Check sheet for the modelled part. Datum: model origin and axes. Units: mm. A direction names the side the tool comes from. Coordinates: 2 decimals unless noted, no trailing zeros. Write each loop counter-clockwise with the first axis right and the second up, starting at its lowest first coordinate (ties: lowest second). Pieces come first, ordered by that corner, then holes. Notation, with made-up numbers: (77, 47.5) -> (108, 47.5) arc R6 cw to (108, 57.5) -> close; hole circle Ø9 at (-28.5, 86.25). An arc over 180 degrees is marked (long way). One line per item, written item: value. Start each with the question number.
1) Sectioned sample at B-B on x = 11.43. Enter the section's corners in (y, z).
2) Gauge pin test, flat ends, axial feed: P1, Ø12, axis at x = 0, y = 0, coming from the -Z side; P2, Ø5.5, axis at x = -23.5, z = -15.5, coming from the -Y side; P3, Ø8, axis at x = -28, y = 19, coming from the +Z side. Record the tip position at first contact, or that the pin passes through.
3) Sectioned sample at C-C on y = -12.7. Enter the section's corners in (x, z).
4) Set-up check for faces 5 (the cylindrical face through (-54.72, 5.79, -8.81)), 6 (the flat face through (-26.513, -15.382, 22.181)), 7 (the flat face through (-35.324, 20.149, -22.269)), 8 (the flat face through (1.27, -24, 16)), 9 (the flat face through (-47.714, 0, -17)): record each of +Z, -Z, +X, -X, +Y, -Y from which the full face is reachable in a straight line by a thin tool's end or side.
5) Sectioned sample at D-D on x = -44.5. Enter the section's corners in (y, z), plus the area to 3 significant figures.
6) Scan lines: line 1 along X through (y, z) = (22, 13); line 2 along Y through (x, z) = (0, -11.25) (3 decimals); line 3 along Z through (x, y) = (20.5, -19). Record each from-to range of solid material in increasing order. Write a range as [from, to].
7) Draft check along Y on faces 1 (the flat face through (-28.354, 20.149, -22.269)), 2 (the cylindrical face through (-31.899, -3.176, -22.269)), 3 (the cylindrical face through (-54.7, 6.4, 8.7)), 4 (the flat face through (0, 0, 25.4)). Enter one of: +Y half, -Y half, draft (parallel to the pull), parting line (faces both ways), or undercut.
8) Sectioned sample at A-A on z = 10.16. Enter the section's corners in (x, y).
Autodesk Inventor part; units mm, degrees
ref_plane "YZ Plane" through (0, 0, 0) normal (1, 0, 0) x (0, 1, 0)
ref_plane "XZ Plane" through (0, 0, 0) normal (0, 1, 0) x (-1, 0, 0)
ref_plane "XY Plane" through (0, 0, 0) normal (0, 0, 1) x (1, 0, 0)
sketch "Sketch1" plane through (0, 0, 0) normal (0, 0, 1) x (1, 0, 0)
  line L0 (-57.8485, 25.4) -> (-51.4985, 25.4)
  line L1 (-51.4985, 25.4) -> (-51.4985, -25.4)
  line L2 (-51.4985, -25.4) -> (-57.8485, -25.4)
  line L3 (-57.8485, -25.4) -> (-57.8485, 25.4)
  line L4 (25.4, 25.4) -> (31.75, 25.4)
  line L5 (31.75, 25.4) -> (31.75, -25.4)
  line L6 (31.75, -25.4) -> (25.4, -25.4)
  line L7 (25.4, -25.4) -> (25.4, 25.4)
  point P0 (0, 0)
  dimension "d0" = 6.35
  dimension "d1" = 50.8
  dimension "d2" = 25.4
  dimension "d3" = 51.4985
  dimension "d4" = 25.4
  dimension "d5" = 25.4
extrude "Extrusion1" add sketch "Sketch1" along normal mid plane 38.1
sketch "Sketch2" plane through (0, 0, 19.05) normal (0, 0, 1) x (1, 0, 0)
  line L0 (-51.4985, 25.4) -> (-57.8485, 25.4)
  line L1 (31.75, -25.4) -> (25.4, -25.4)
  line L2 (-57.8485, 25.4) -> (31.75, 25.4)
  line L3 (31.75, 25.4) -> (31.75, -25.4)
  line L4 (31.75, -25.4) -> (-57.8485, -25.4)
  line L5 (-57.8485, -25.4) -> (-57.8485, 25.4)
  circle A0 centre (0, 0) radius 6.604
  circle A1 centre (-41.3385, 6.35) radius 1.4605
  line L6 (-47.9108, 0) -> (-31.2118, 0) construction
  circle A2 centre (-41.3385, -6.35) radius 1.4605
  line L7 (-51.4985, -25.4) -> (-51.4985, 25.4)
  dimension "d8" = 13.208
  dimension "d40" = 2.921
  dimension "d42" = 19.05
  dimension "d43" = 16.51
  dimension "d44" = 6.35
  dimension "d92" = 6.35
sketch "Sketch3" plane through (0, 0, -19.05) normal (0, 0, -1) x (-1, 0, 0)
  line L0 (-31.75, 25.4) -> (-31.75, -25.4)
  line L1 (51.4985, -25.4) -> (57.8485, -25.4)
  line L2 (-31.75, 25.4) -> (57.8485, 25.4)
  line L3 (57.8485, 25.4) -> (57.8485, -25.4)
  line L4 (57.8485, -25.4) -> (-31.75, -25.4)
  line L5 (-31.75, -25.4) -> (-31.75, 25.4)
  circle A0 centre (0, 0) radius 6.604
  circle A1 centre (-11.43, 0.0226) radius 2.54
  circle A2 centre (-20.2438, 8.7122) radius 1.7907
  line L6 (-13.9699, 0) -> (6.604, 0) construction
  circle A3 centre (-20.2438, -8.7122) radius 1.7907
  circle A4 centre (41.3385, 6.35) radius 1.4605
  line L7 (51.4985, 25.4) -> (51.4985, -25.4)
  circle A5 centre (41.3385, -6.35) radius 1.4605
  dimension "d11" = 13.208
  dimension "d12" = 5.08
  dimension "d13" = 11.43
  dimension "d14" = 3.5814
  dimension "d15" = 20.2438
  dimension "d16" = 8.7122
  dimension "d32" = 2.921
  dimension "d33" = 10.16
  dimension "d34" = 6.35
  dimension "d35" = 6.35
extrude "Extrusion7" add sketch "Sketch2" along normal blind 6.35
extrude "Extrusion6" add sketch "Sketch3" along normal blind 6.35
sketch "Sketch6" plane through (-57.8485, -25.4, 25.4) normal (-1, 0, 0) x (0, 0, 1)
  circle A0 centre (-23.114, 38.1) radius 1.4605
  line L0 (-35.0625, 25.4) -> (-10.5897, 25.4) construction
  line L1 (0, 0) -> (-50.8, 0) construction
  line L2 (0, 50.8) -> (0, 0) construction
  circle A1 centre (-23.114, 12.7) radius 1.4605
  point P0 (-25.4, 25.4)
  dimension "d47" = 2.921
  dimension "d48" = 25.4
  dimension "d49" = 12.7
  dimension "d50" = 23.114
extrude "Extrusion8" cut sketch "Sketch6" against normal up to next
sketch "Sketch8" plane through (-57.8485, 25.4, 25.4) normal (0, 1, 0) x (1, 0, 0)
  line L0 (0, 50.8) -> (0, 0)
  line L1 (0, 21.59) -> (6.35, 21.59)
  line L2 (6.35, 21.59) -> (6.35, 29.21)
  line L3 (6.35, 29.21) -> (0, 29.21)
  line L4 (0, 29.21) -> (0, 21.59)
  line L5 (0, 25.4) -> (6.35, 25.4) construction
  line L6 (89.5985, 0) -> (0, 0)
  line L7 (0, 50.8) -> (89.5985, 50.8)
  line L8 (6.35, 6.35) -> (6.35, 44.45)
  point P0 (57.8485, 25.4)
  point P1 (0, 29.21)
  dimension "d56" = 25.4
  dimension "d57" = 50.8
  dimension "d58" = 7.62
extrude "Extrusion10" cut sketch "Sketch8" against normal through all
sketch "Sketch10" plane through (0, 0, 25.4) normal (0, 0, 1) x (1, 0, 0)
  circle A0 centre (20.2438, -8.7122) radius 1.7907 construction
  circle A1 centre (20.2438, -8.7122) radius 1.7907
  circle A2 centre (20.2438, 8.7122) radius 1.7907 construction
  circle A3 centre (20.2438, 8.7122) radius 1.7907
  circle A4 centre (20.2438, 8.7122) radius 5.08
  circle A5 centre (20.2438, -8.7122) radius 5.08
  point P0 (0, 0)
  dimension "d64" = 10.16
extrude "Extrusion12" cut sketch "Sketch10" against normal blind 25.4 contours A1 | A3 | A4 | A5
sketch "Sketch11" plane through (0, 0, 25.4) normal (0, 0, 1) x (1, 0, 0)
  line L0 (9.525, -9.525) -> (-9.525, -9.525)
  line L1 (-9.525, -9.525) -> (-9.525, 9.525)
  line L2 (-9.525, 9.525) -> (9.525, 9.525)
  line L3 (9.525, 9.525) -> (9.525, -9.525)
  line L4 (9.525, -9.525) -> (-9.525, 9.525) construction
  line L5 (-9.525, -9.525) -> (9.525, 9.525) construction
  point P0 (0, 0)
  dimension "d67" = 19.05
  dimension "d68" = 19.05
extrude "Extrusion13" add sketch "Sketch11" along normal blind 6.35
sketch "Sketch12" plane through (0, 0, -25.4) normal (0, 0, -1) x (-1, 0, 0)
  circle A0 centre (31.8389, -6.35) radius 3.175
  line L0 (57.8485, -25.4) -> (57.8485, 25.4)
  line L1 (34.9338, -5.6412) -> (39.4589, -25.4)
  line L2 (28.744, -5.6412) -> (24.2189, -25.4)
  line L3 (24.2189, -25.4) -> (39.4589, -25.4)
  line L4 (-25.4, -25.4) -> (51.4985, -25.4)
  circle A1 centre (31.8389, 15.24) radius 3.175
  line L5 (57.8485, 25.4) -> (-31.75, 25.4)
  line L6 (28.67, 15.0438) -> (28.0289, 25.4)
  line L7 (51.4985, 25.4) -> (-25.4, 25.4)
  line L8 (35.0078, 15.0438) -> (35.6489, 25.4)
  point P0 (0, 0)
  dimension "d71" = 6.35
  dimension "d72" = 26.0096
  dimension "d73" = 6.35
  dimension "d74" = 15.24
  dimension "d75" = 7.62
  dimension "d78" = 10.16
  dimension "d79" = 7.62
  dimension "d80" = 3.81
extrude "Extrusion14" cut sketch "Sketch12" against normal through all
sketch "Sketch13" plane through (0, 0, -19.05) normal (0, 0, 1) x (1, 0, 0)
  circle A0 centre (0, 0) radius 6.604
  circle A1 centre (0, 0) radius 6.604
  circle A2 centre (0, 0) radius 9.525
  dimension "d81" = 19.05
extrude "Extrusion15" add sketch "Sketch13" along normal blind 12.192
sketch "Sketch14" plane through (31.75, 25.4, 25.4) normal (0, 1, 0) x (1, 0, 0)
  line L0 (-59.7789, 50.8) -> (0, 50.8)
  line L1 (-22.225, 0) -> (-41.275, 0)
  line L2 (-40.64, 50.8) -> (-30.48, 50.8)
  line L3 (-30.48, 50.8) -> (-30.48, 0)
  line L4 (-30.48, 0) -> (-40.64, 0)
  line L5 (-40.64, 0) -> (-40.64, 50.8)
  line L6 (0, 0) -> (0, 50.8)
  point P0 (-31.75, 25.4)
  dimension "d84" = 10.16
  dimension "d85" = 40.64
extrude "Extrusion16" add sketch "Sketch14" against normal blind 3.81
sketch "Sketch15" plane through (0, 0, 19.05) normal (0, 0, -1) x (-1, 0, 0)
  circle A0 centre (0, 0) radius 9.525
  circle A1 centre (0, 0) radius 6.604
extrude "Extrusion17" add sketch "Sketch15" along normal blind 5.08
sketch "Sketch16" plane through (31.75, -25.4, -25.4) normal (0, -1, 0) x (1, 0, 0)
  line L0 (-40.64, 44.45) -> (-30.48, 44.45)
  line L1 (-40.64, 44.45) -> (-40.64, 6.35)
  line L2 (-30.48, 6.35) -> (-40.64, 6.35)
  line L3 (-30.48, 6.35) -> (-30.48, 44.45)
  point P0 (-31.75, 25.4)
extrude "Extrusion18" add sketch "Sketch16" against normal blind 3.81
sketch "Sketch17" plane through (0, 0, 25.4) normal (0, 0, 1) x (1, 0, 0)
  arc A0 (-35.0078, 15.0438) -> (-28.67, 15.0438) centre (-31.8389, 15.24) ccw construction
  line L0 (-31.8389, 12.065) -> (-31.8389, -3.175) construction
  arc A1 (-28.744, -5.6412) -> (-34.9338, -5.6412) centre (-31.8389, -6.35) ccw construction
  circle A2 centre (-41.3385, 6.35) radius 1.4605
  circle A3 centre (-41.3385, 6.35) radius 1.4605
  circle A4 centre (-22.3393, 6.35) radius 1.4605
  point P0 (0, 0)
extrude "Extrusion19" cut sketch "Sketch17" against normal through all contours A4
sketch "Sketch19" plane through (-57.8485, -25.4, -25.4) normal (-1, 0, 0) x (0, 0, 1)
  circle A0 centre (15.24, 31.75) radius 1.4605
  circle A1 centre (15.24, 19.05) radius 1.4605
  line L0 (21.59, 0) -> (21.59, 50.8) construction
  line L1 (0, 50.8) -> (21.59, 50.8) construction
  line L2 (25.4, 25.4) -> (25.4, 50.8) construction
  line L3 (6.35, 50.8) -> (44.45, 50.8) construction
  circle A2 centre (35.56, 31.75) radius 1.4605
  circle A3 centre (35.56, 19.05) radius 1.4605
  dimension "d95" = 6.35
  dimension "d96" = 2.921
  dimension "d97" = 2.921
  dimension "d98" = 12.7
  dimension "d99" = 19.05
extrude "Extrusion20" cut sketch "Sketch19" against normal blind 12.7
sketch "Sketch20" plane through (31.75, -25.4, 25.4) normal (1, 0, 0) x (0, 0, -1)
  circle A0 centre (25.4, 38.1) radius 2.4384
  circle A1 centre (25.4, 12.7) radius 2.4384
  line L0 (50.8, 50.8) -> (50.8, 0)
  line L1 (0, 0) -> (0, 50.8)
  line L2 (0, 50.8) -> (50.8, 50.8)
  point P0 (25.4, 25.4)
  dimension "d102" = 25.4
  dimension "d103" = 50.8
  dimension "d104" = 25.4
  dimension "d105" = 12.7
  dimension "d106" = 4.8768
extrude "Extrusion21" cut sketch "Sketch20" against normal blind 25.4
sketch "Sketch21" plane through (0, 0, -19.05) normal (0, 0, 1) x (1, 0, 0)
  circle A0 centre (-22.3393, 6.35) radius 1.4605
  line L0 (1.27, -21.59) -> (1.27, -25.4)
  line L1 (25.4, -25.4) -> (1.27, -25.4)
  line L2 (25.4, -25.4) -> (25.4, 25.4)
  line L3 (1.27, 25.4) -> (25.4, 25.4)
  line L4 (1.27, 25.4) -> (1.27, 21.59)
  line L5 (1.27, 21.59) -> (-8.89, 21.59)
  line L6 (-8.89, 21.59) -> (-8.89, 25.4)
  line L7 (-28.0289, 25.4) -> (-8.89, 25.4)
  line L8 (-28.0289, 25.4) -> (-28.67, 15.0438)
  arc A1 (-35.0078, 15.0438) -> (-28.67, 15.0438) centre (-31.8389, 15.24) ccw
  line L9 (-35.0078, 15.0438) -> (-35.6489, 25.4)
  line L10 (-51.4985, 25.4) -> (-35.6489, 25.4)
  line L11 (-51.4985, 25.4) -> (-51.4985, -25.4)
  line L12 (-39.4589, -25.4) -> (-51.4985, -25.4)
  line L13 (-39.4589, -25.4) -> (-34.9338, -5.6412)
  arc A2 (-28.744, -5.6412) -> (-34.9338, -5.6412) centre (-31.8389, -6.35) ccw
  line L14 (-28.744, -5.6412) -> (-24.2189, -25.4)
  line L15 (-8.89, -25.4) -> (-24.2189, -25.4)
  line L16 (-8.89, -25.4) -> (-8.89, -21.59)
  line L17 (-8.89, -21.59) -> (1.27, -21.59)
  circle A3 centre (20.2438, -8.7122) radius 1.7907
  circle A4 centre (20.2438, 8.7122) radius 1.7907
  circle A5 centre (-41.3385, -6.35) radius 1.4605
  circle A6 centre (-41.3385, 6.35) radius 1.4605
  arc A7 (9.3985, 1.5472) -> (9.4045, -1.5101) centre (0, 0) ccw
  arc A8 (9.4045, -1.5101) -> (9.3985, 1.5472) centre (11.43, 0.0226) ccw
  line L18 (-47.7139, 10.16) -> (-15.9639, 10.16)
  line L19 (-15.9639, 10.16) -> (-15.9639, -10.16)
  line L20 (-15.9639, -10.16) -> (-47.7139, -10.16)
  line L21 (-47.7139, -10.16) -> (-47.7139, 10.16)
  point P0 (-27.7091, -10.16)
  point P1 (-35.9687, -10.16)
  dimension "d109" = 6.3754
  dimension "d110" = 31.75
  dimension "d111" = 20.32
  dimension "d112" = 10.16
extrude "Extrusion22" add sketch "Sketch21" along normal blind 4.953 contours L14 A2 L13 L20 L21 L18 L19
sketch "Sketch22" plane through (31.75, -25.4, -25.4) normal (0, -1, 0) x (1, 0, 0)
  line L0 (-40.64, 6.35) -> (-40.64, 44.45)
  line L1 (-40.64, 18.3213) -> (-30.446, 18.3213)
  line L2 (-30.446, 18.3213) -> (-30.446, 37.9181)
  line L3 (-30.446, 37.9181) -> (-40.64, 37.9181)
  line L4 (-40.64, 37.9181) -> (-40.64, 18.3213)
  point P0 (-31.75, 25.4)
  point P1 (-40.64, 37.9181)
extrude "Extrusion23" cut sketch "Sketch22" against normal blind 6.35
equation "\"d56\" = 0.5 * d57"
equation "\"d75\" = 0.5 * d74"
equation "\"d80\" = 0.5 * d79"
equation "\"d102\" = 0.5 * d103"
equation "\"d107\" = d104"
properties part number "NewCasing"
Answers:
1. outline: (-25.4, -25.4) -> (-2.52, -25.4) -> (-2.52, -19.05) -> (-25.4, -19.05) -> close; (-25.4, 19.05) -> (25.4, 19.05) -> (25.4, 25.4) -> (-25.4, 25.4) -> close; (2.56, -25.4) -> (25.4, -25.4) -> (25.4, -19.05) -> (2.56, -19.05) -> close
2. P1: stops at z = 25.4
2. P2: stops at y = -10.16
2. P3: stops at z = 25.4
3. outline: (-57.85, -25.4) -> (-36.55, -25.4) -> (-36.55, -19.05) -> (-51.5, -19.05) -> (-51.5, -3.81) -> (-57.85, -3.81) -> close; (-57.85, 3.81) -> (-51.5, 3.81) -> (-51.5, 19.05) -> (-36.55, 19.05) -> (-36.55, 25.4) -> (-57.85, 25.4) -> close; (-27.13, -25.4) -> (31.75, -25.4) -> (31.75, -2.44) -> (25.4, -2.44) -> (25.4, -19.05) -> (-27.13, -19.05) -> close; (-27.13, 19.05) -> (17.1, 19.05) -> (17.1, 25.4) -> (-27.13, 25.4) -> close; (23.39, 19.05) -> (25.4, 19.05) -> (25.4, 2.44) -> (31.75, 2.44) -> (31.75, 25.4) -> (23.39, 25.4) -> close
4. face 5: -X
4. face 6: +Z, -Z, -Y
4. face 7: +Z, -Z, +Y
4. face 8: -Y
4. face 9: +Y, -Y
5. outline: (-25.4, -25.4) -> (25.4, -25.4) -> (25.4, -19.05) -> (10.16, -19.05) -> (10.16, -14.1) -> (-10.16, -14.1) -> (-10.16, -19.05) -> (-25.4, -19.05) -> close; (-25.4, 19.05) -> (25.4, 19.05) -> (25.4, 25.4) -> (-25.4, 25.4) -> close
5. area: 746 mm2
6. line 1: x = [-57.85, -51.5], [-8.89, 1.27], [25.4, 31.75]
6. line 2: y = [-25.4, -21.59], [-9.525, -6.604], [6.604, 9.525], [21.59, 25.4]
6. line 3: z = [-25.4, -19.05], [19.05, 25.4]
7. face 1: +Y half
7. face 2: -Y half
7. face 3: undercut
7. face 4: undercut
8. outline: (-57.85, -25.4) -> (-51.5, -25.4) -> (-51.5, -7.81) -> (-57.85, -7.81) -> close; (-57.85, -4.89) -> (-51.5, -4.89) -> (-51.5, 4.89) -> (-57.85, 4.89) -> close; (-57.85, 7.81) -> (-51.5, 7.81) -> (-51.5, 25.4) -> (-57.85, 25.4) -> close; (-8.89, 21.59) -> (1.27, 21.59) -> (1.27, 25.4) -> (-8.89, 25.4) -> close; (25.4, -25.4) -> (31.75, -25.4) -> (31.75, 25.4) -> (25.4, 25.4) -> close
